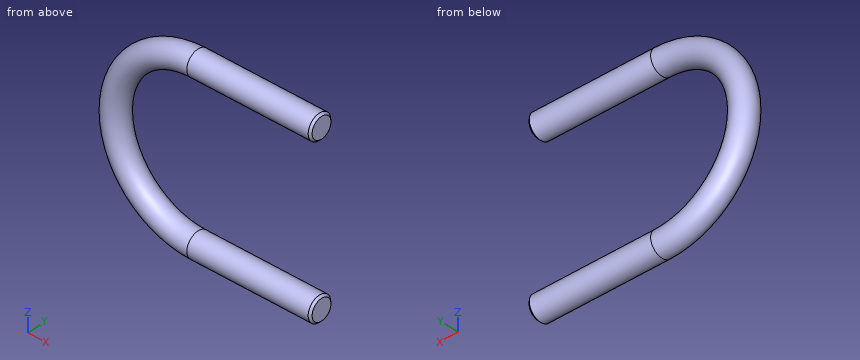
Autodesk Inventor part; units mm, degrees
ref_plane "YZ Plane" through (0, 0, 0) normal (1, 0, 0) x (0, 1, 0)
ref_plane "XZ Plane" through (0, 0, 0) normal (0, 1, 0) x (-1, 0, 0)
ref_plane "XY Plane" through (0, 0, 0) normal (0, 0, 1) x (1, 0, 0)
sketch "Esboço1" plane through (0, 0, 0) normal (1, 0, 0) x (0, 1, 0)
  line L0 (0, 0) -> (15, 0)
  circle A0 centre (0, -20) radius 3
revolve "Revolução1" add sketch "Esboço1" angle 180 about axis through (0, 0, 0) along (0, 1, 0)
sketch "Esboço2" plane through (0, 0, 20) normal (1, 0, 0) x (0, 0, -1)
  circle A0 centre (0, 0) radius 3
  circle A1 centre (40, 0) radius 3
  point P0 (20, 0)
extrude "Extrusão1" add sketch "Esboço2" along normal blind 30
chamfer "Chanfro1" distance 0.5 angle 45 2 edges at (30, 0, -17) (30, 0, 23)
sketch "Esboço3" plane through (0, 0, 0) normal (0, 1, 0) x (-1, 0, 0)
  point P0 (0, 0)
thread "Rosca1"
thread "Rosca2"
properties part number "parafuso u abraçadeira" material "Aço inoxidável"
CAD build for the part. Positions are in the model's coordinates, mm. Give positions to 0.01 mm unless a question says otherwise; leave off trailing zeros. Order: outer loops, then holes, each group sorted by start corner. A loop starts at its lowest first (then second) coordinate and runs counter-clockwise, first axis right, second up. Notation, with made-up numbers: M 64,-2 L 97,-2 A24 ccw 97,22 Z; hole C 18.25,9.25 d4. An arc over 180 degrees is marked long. Put each result on its own line as item: value. Start each with the question number.
(1) Flat gauge pins, fed straight in: pin 1 Ø1.5 at (x, y) = (-16.5, -1) entering from +Z; pin 2 Ø3 at (y, z) = (0, -1) entering from -X; pin 3 Ø1.5 at (x, z) = (3.5, -18) entering from -Y. Where does each tip first touch, or does it go through?
(2) Saw through at A-A, the plane x = 13. Write the cut outline in (y, z), then the cut area to 3 significant figures.
(3) Drill centre lines: line 1 along Z through (x, y) = (7, 0.25); line 2 along Z through (x, y) = (28.5, -1.25); line 3 along X through (y, z) = (-2.5, -10.5). Where is each one in solid material? Low to high.
(4) Saw through at B-B, the plane y = 0. Write the cut outline in (x, z).
Check result:
1. pin 1: stops at z = 16.59
1. pin 2: stops at x = -23
1. pin 3: stops at y = -2.73
2. outline: C 0,-20 d6; C 0,20 d6
2. area: 56.5 mm2
3. line 1: z = -22.99 to -17.01, 17.01 to 22.99
3. line 2: z = -22.73 to -17.27, 17.27 to 22.73
3. line 3: x = -18.94 to -15.04
4. outline: M 0,-23 L 29.5,-23 L 30,-22.5 L 30,-17.5 L 29.5,-17 L 0,-17 A17 cw 0,17 L 29.5,17 L 30,17.5 L 30,22.5 L 29.5,23 L 0,23 A23 ccw Z
